```python
from build123d import *

# Parameters (mm, degrees)
ESQUISSE1_W                     = 360
ESQUISSE1_H                     = 330
BOSS_EXTRU_1_DEPTH              = 1.5
ESQUISSE2_R                     = 5
ENL_V_MAT_EXTRU_1_DEPTH         = 1.5
BOSS_EXTRU_2_START              = 1
ESQUISSE3_R                     = 7
ESQUISSE3_R_2                   = 5
BOSS_EXTRU_2_DEPTH              = 1
CONG_2_R                        = 8
CONG_4_R                        = 8
R_P_TITION_LIN_AIRE2_COUNT      = 2
R_P_TITION_LIN_AIRE2_PITCH      = 343
R_P_TITION_LIN_AIRE2_COUNT_DIR2 = 2
R_P_TITION_LIN_AIRE2_PITCH_DIR2 = 314
ENL_V_MAT_EXTRU_2_DEPTH         = 0.2
ENL_V_MAT_EXTRU_3_DEPTH         = 0.2
BOSS_EXTRU_3_DEPTH              = 0.2
BOSS_EXTRU_4_DEPTH              = 0.2
BOSS_EXTRU_5_DEPTH              = 0.2
ESQUISSE9_W                     = 40
ESQUISSE9_H                     = 40
BOSS_EXTRU_6_DEPTH              = 10


with BuildPart() as part:
    # Esquisse1 → Boss.-Extru.1 (new body)
    with BuildSketch(Plane.XY):
        with Locations((-180, 165)):
            Rectangle(ESQUISSE1_W, ESQUISSE1_H)
    extrude(amount=BOSS_EXTRU_1_DEPTH)

    # Esquisse2 → Enlèv. mat.-Extru.1 (cut)
    with BuildSketch(Plane.XY.offset(1.5)):
        with Locations((-352, 322)):
            Circle(ESQUISSE2_R)
    enl_v_mat_extru_1 = extrude(amount=-ENL_V_MAT_EXTRU_1_DEPTH, mode=Mode.SUBTRACT)

    # Esquisse3 → Boss.-Extru.2 (add)
    with BuildSketch(Plane.XY.offset(1.5).offset(BOSS_EXTRU_2_START)):
        with Locations((-352, 322)):
            Circle(ESQUISSE3_R)
        with Locations((-352, 322)):
            Circle(ESQUISSE3_R_2, mode=Mode.SUBTRACT)
    boss_extru_2 = extrude(amount=-BOSS_EXTRU_2_DEPTH)

    # Congé2
    cong_2_edges = [part.edges().sort_by_distance(p)[0] for p in [
        (-360, 0, 0.75),
        (-360, 330, 0.75),
    ]]
    fillet(cong_2_edges, radius=CONG_2_R)

    # Congé4
    cong_4_edges = [part.edges().sort_by_distance(p)[0] for p in [
        (0, 0, 0.75),
        (0, 330, 0.75),
    ]]
    fillet(cong_4_edges, radius=CONG_4_R)

    # Répétition linéaire2: Enlèv. mat.-Extru.1, Boss.-Extru.2 2 × 2
    with Locations(*[(i * R_P_TITION_LIN_AIRE2_PITCH, -j * R_P_TITION_LIN_AIRE2_PITCH_DIR2, 0) for i in range(R_P_TITION_LIN_AIRE2_COUNT) for j in range(R_P_TITION_LIN_AIRE2_COUNT_DIR2) if (i, j) != (0, 0)]):
        add(enl_v_mat_extru_1, mode=Mode.SUBTRACT)
        add(boss_extru_2)

    # Esquisse4 → Enlèv. mat.-Extru.2 (cut)
    with BuildSketch(Plane.XY.offset(1.5)):
        Polygon((-342.224801163, 320), (-18.072831487, 320), (-10, 311.927168513), (-10, 16.768229134), (-18.072831487, 10), (-343.231770866, 10), (-350, 16.768229134), (-350, 312.224801163), align=None)
    extrude(amount=-ENL_V_MAT_EXTRU_2_DEPTH, mode=Mode.SUBTRACT)

    # Esquisse5 → Enlèv. mat.-Extru.3 (cut)
    with BuildSketch(Plane.XY.offset(1.3)):
        Polygon((-180, 155), (-170, 165), (-180, 175), (-190, 165), align=None)
    extrude(amount=-ENL_V_MAT_EXTRU_3_DEPTH, mode=Mode.SUBTRACT)

    # Esquisse6 → Boss.-Extru.3 (add)
    with BuildSketch(Plane.XY.offset(1.3)):
        Polygon((-190.148829514, 320), (-180.16505775, 310.000013168), (-170.148829514, 320), align=None)
        Polygon((-350, 174.492138197), (-340, 164.492138197), (-350, 154.492138197), align=None)
        Polygon((-190.285016954, 8.853157765), (-180.292495127, 18.844401072), (-170.285024617, 8.835649966), align=None)
    extrude(amount=BOSS_EXTRU_3_DEPTH)

    # Esquisse7 → Boss.-Extru.4 (add)
    with BuildSketch(Plane.XY.offset(1.3)):
        Polygon((-10, 175), (-20, 165), (-10, 155), align=None)
    extrude(amount=BOSS_EXTRU_4_DEPTH)

    # Esquisse8 → Boss.-Extru.5 (add)
    with BuildSketch(Plane.XY.offset(1.3)):
        Polygon((-341, 163.492138197), (-188.492138197, 163.492138197), (-190, 165), (-189.507861803, 165.492138197), (-341, 165.492138197), align=None)
        Polygon((-6.914170883, 165.492138197), (-6.914170883, 163.492138197), (-171.507861803, 163.492138197), (-170, 165), (-170.492138197, 165.492138197), align=None)
    extrude(amount=BOSS_EXTRU_5_DEPTH)

    # Esquisse9 → Boss.-Extru.6 (add)
    with BuildSketch(Plane(origin=(0, 0, 0), x_dir=(-1, 0, 0), z_dir=(0, 0, -1))):
        with Locations((25, 165)):
            Rectangle(ESQUISSE9_W, ESQUISSE9_H)
    extrude(amount=BOSS_EXTRU_6_DEPTH)


solid = part.part
```
CAD build for the part. Positions are in the model's coordinates, mm. A direction names the side the tool comes from. Round coordinates to 2 decimals unless told otherwise and drop trailing zeros. Write each loop counter-clockwise with the first axis right and the second up, starting at its lowest first coordinate (ties: lowest second). Pieces come first, ordered by that corner, then holes.
Item 1: Drop flat-ended pins along their axis: pin 1 Ø6 at (x, y) = (-185.5, 130) entering from +Z; pin 2 Ø3 at (x, y) = (-244.5, 104) entering from -Z; pin 3 Ø5 at (x, z) = (-29.5, -3) entering from +Y. Give the stop position or say it passes through.
Filled in:
pin 1: stops at z = 1.3
pin 2: stops at z = 0
pin 3: stops at y = 185
Item 2: Tool access for faces 1 (the flat face through (-180, 165, 1.1)), 2 (the flat face through (-25, 145, -5)): list every direction of +Z, -Z, +X, -X, +Y, -Y with a clear straight run to the whole face (end or side of a thin tool).
Filled in:
face 1: +Z
face 2: -Z, +X, -X, -Y
Item 3: Drill centre lines: L1, parallel to X at y = 322, z = 1.6; L2, parallel to Y at x = -352, z = 1.6; L3, parallel to Y at x = -9, z = 1.15. Where is each one in solid material? Low to high.
Filled in:
L1: x = -359 to -357, -347 to -345, -16 to -14, -4 to -2
L2: y = 1 to 3, 13 to 15, 315 to 317, 327 to 329
L3: y = 0 to 3, 13 to 317, 327 to 330
Item 4: Band-saw the part on A-A on y = 35. Write the cut outline in (x, z), then the cut area to 3 significant figures.
Filled in:
outline: (-360, 0) - (0, 0) - (0, 1.5) - (-10, 1.5) - (-10, 1.3) - (-350, 1.3) - (-350, 1.5) - (-360, 1.5) - close
area: 472 mm2
Item 5: Band-saw the part on B-B on x = -316. Write the cut outline in (y, z), then the cut area to 3 significant figures.
Filled in:
outline: (0, 0) - (330, 0) - (330, 1.5) - (320, 1.5) - (320, 1.3) - (165.49, 1.3) - (165.49, 1.5) - (163.49, 1.5) - (163.49, 1.3) - (10, 1.3) - (10, 1.5) - (0, 1.5) - close
area: 433 mm2
Item 6: Band-saw the part on C-C on z = -3.25. Write the cut outline in (x, y).
Filled in:
outline: (-45, 145) - (-5, 145) - (-5, 185) - (-45, 185) - close
Item 7: Band-saw the part on D-D on y = 179. Write the cut outline in (x, z).
Filled in:
outline: (-360, 0) - (-45, 0) - (-45, -10) - (-5, -10) - (-5, 0) - (0, 0) - (0, 1.5) - (-10, 1.5) - (-10, 1.3) - (-350, 1.3) - (-350, 1.5) - (-360, 1.5) - close
